```python
from build123d import *

# Parameters (mm, degrees)
SKETCH1_R           = 4.5
SKETCH1_R_2         = 3.175
BOSS_EXTRUDE1_DEPTH = 6.35


with BuildPart() as part:
    # Sketch1 → Boss-Extrude1 (new body)
    with BuildSketch(Plane.XY):
        with BuildLine():
            Line((-88.9, 6.35), (88.9, 6.35))
            ThreePointArc((88.9, 6.35), (95.25, 0), (88.9, -6.35))
            Line((88.9, -6.35), (-88.9, -6.35))
            ThreePointArc((-88.9, -6.35), (-95.25, 0), (-88.9, 6.35))
        make_face()
        with Locations((-88.9, 0)):
            Circle(SKETCH1_R, mode=Mode.SUBTRACT)
        with Locations((88.9, 0)):
            Circle(SKETCH1_R, mode=Mode.SUBTRACT)
        Circle(SKETCH1_R_2, mode=Mode.SUBTRACT)
    extrude(amount=BOSS_EXTRUDE1_DEPTH)


solid = part.part
```
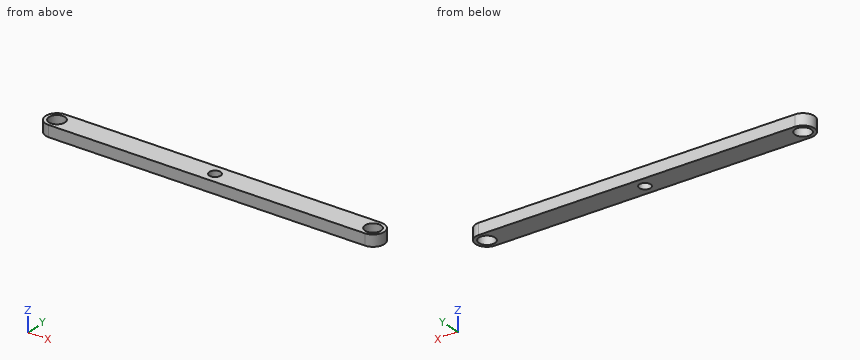
Input: part model. Units: mm. Frame: model coordinates. Coordinates: 2 decimals unless noted, no trailing zeros. Write each loop counter-clockwise with the first axis right and the second up, starting at its lowest first coordinate (ties: lowest second). Pieces come first, ordered by that corner, then holes. Notation, with made-up numbers: M -21,58 L -4,58 A14 cw -4,75 Z; hole C 50,-39.5 d9. An arc over 180 degrees is marked long. Use one line per item in the form item = value.
Q1. Material intervals for probe 1 along X at (y, z) = (-3.5, 4); probe 2 along X at (y, z) = (-2, 2.25); probe 3 along X at (y, z) = (-4, 4.25), sorted ascending. Write a range as from..to.
Answer below:
probe_1 = -94.2..-91.73, -86.07..86.07, 91.73..94.2
probe_2 = -94.93..-92.93, -84.87..-2.47, 2.47..84.87, 92.93..94.93
probe_3 = -93.83..-90.96, -86.84..86.84, 90.96..93.83
Q2. Section A-A (y = 0). Return loops of the section in (x, z) (3 decimals).
Answer below:
outline = M -95.25,0 L -93.4,0 L -93.4,6.35 L -95.25,6.35 Z; M -84.4,0 L -3.175,0 L -3.175,6.35 L -84.4,6.35 Z; M 3.175,0 L 84.4,0 L 84.4,6.35 L 3.175,6.35 Z; M 93.4,0 L 95.25,0 L 95.25,6.35 L 93.4,6.35 Z
Q3. Section B-B (z = 1). Return loops of the section in (x, y) (3 decimals), plus the area to 3 significant figures.
Answer below:
outline = M -88.9,-6.35 L 88.9,-6.35 A6.35 ccw 88.9,6.35 L -88.9,6.35 A6.35 ccw Z; hole C -88.9,0 d9; hole C 0,0 d6.35; hole C 88.9,0 d9
area = 2,230 mm²
Q4. Section C-C (x = 0). Return loops of the section in (y, z) (3 decimals), plus the area to 3 significant figures.
Answer below:
outline = M -6.35,0 L -3.175,0 L -3.175,6.35 L -6.35,6.35 Z; M 3.175,0 L 6.35,0 L 6.35,6.35 L 3.175,6.35 Z
area = 40.3 mm²
